from build123d import *

# Parameters (mm, degrees)
SKETCH2_W          = 23
SKETCH2_H          = 23.33
BASE_FLANGE1_DEPTH = 1.17
FILLET1_R          = 5


# Sheet-metal steps are written as plain solids
with BuildPart() as part:
    # Sketch2 → Base-Flange1 (new body)
    with BuildSketch(Plane.XY):
        with Locations((11.5, 11.665)):
            Rectangle(SKETCH2_W, SKETCH2_H)
    extrude(amount=-BASE_FLANGE1_DEPTH)

    # Fillet1
    fillet1_edges = [part.edges().sort_by_distance(p)[0] for p in [
        (0, 23.33, -0.585),
        (23, 23.33, -0.585),
        (23, 0, -0.585),
        (0, 0, -0.585),
    ]]
    fillet(fillet1_edges, radius=FILLET1_R)


solid = part.part
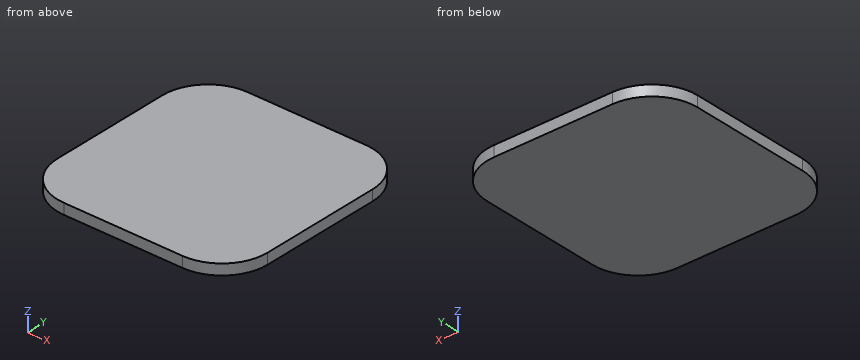
Here's how the part is built. I have some questions about the finished solid (model axes, mm). Coordinates: 2 decimals unless noted, no trailing zeros. Order: outer loops, then holes, each group sorted by start corner. A loop starts at its lowest first (then second) coordinate and runs counter-clockwise, first axis right, second up.
Item 1: If we section it at C-C on x = 2.5: List the corners of the cut face in (y, z) for me.
Result sheet:
outline: (0.67, -1.17) - (22.66, -1.17) - (22.66, 0) - (0.67, 0) - close
Item 2: If we section it at A-A on z = -0.55: List the corners of the cut face in (x, y) for me.
Result sheet:
outline: (0, 5) arc R5 ccw to (5, 0) - (18, 0) arc R5 ccw to (23, 5) - (23, 18.33) arc R5 ccw to (18, 23.33) - (5, 23.33) arc R5 ccw to (0, 18.33) - close
Item 3: For P1, Ø8, axis at x = 18.5, y = 18.5, coming from the +Z side, with a flat end and sliding along its axis, tell me the tip position at first contact or that it passes through.
Result sheet:
P1: stops at z = 0
Item 4: If we section it at B-B on y = 2: List the corners of the cut face in (x, z) for me.
Result sheet:
outline: (1, -1.17) - (22, -1.17) - (22, 0) - (1, 0) - close
Item 5: I need wall thicknesses on line 1 (Y direction, x = 1.25, z = -0.25); line 2 (Y direction, x = 18.5, z = -0.9); line 3 (X direction, y = 1.5, z = -0.35). Which ranges of each line are inside material? Lowest first, please.
Result sheet:
line 1: y = 1.69 to 21.64
line 2: y = 0.03 to 23.3
line 3: x = 1.43 to 21.57
